Drawing for the job (mm, zero at the part's lowest x, y, z). A direction names the side the tool comes from. Round coordinates to 2 decimals unless told otherwise and drop trailing zeros. Write each loop counter-clockwise with the first axis right and the second up, starting at its lowest first coordinate (ties: lowest second). Pieces come first, ordered by that corner, then holes. Notation, with made-up numbers: M 62,62.25 L 83,62.25 A14 ccw 83,80.25 Z; hole C 81.25,27.25 d6. An arc over 180 degrees is marked long. Use a Markdown table: item, result. Add a question column.
1) Drop flat-ended pins along their axis: P1, Ø2, axis at x = 26.5, y = 25.5, coming from the +Z side; P2, Ø10, axis at y = 15.5, z = 14, coming from the +X side; P3, Ø0.6, axis at y = 23.5, z = 13.5, coming from the -X side. Give the stop position or say it passes through.
2) Slice it at D-D on z = 7.25. Write the cut outline in (x, y).
3) Wall check: probe 1 along Y at (x, z) = (46, 2.5); probe 2 along X at (y, z) = (10, 5.5); probe 3 along X at (y, z) = (15.5, 6.25). Give the ranges that are in metal, low to high.
4) Slice it at B-B on y = 14.25. Write the cut outline in (x, z), plus the area to 3 significant figures.
5) Which spindle directions (+Z, -Z, +X, -X, +Y, -Y) get a long thin tool onto all of the face, cutting with end or side? Do the marked faces 1, 2, 3, 4 and 5. Say none if no direction does.
6) Two-plate mould, pull along X, no slides. Class the marked faces 6, 7 and 8: released by +X, released by -X, zero draft, split by the parting line, or undercut.
7) Slice it at C-C on x = 42. Write the cut outline in (y, z).
8) Slice it at A-A on x = 60. Write the cut outline in (y, z), plus the area to 3 significant figures.
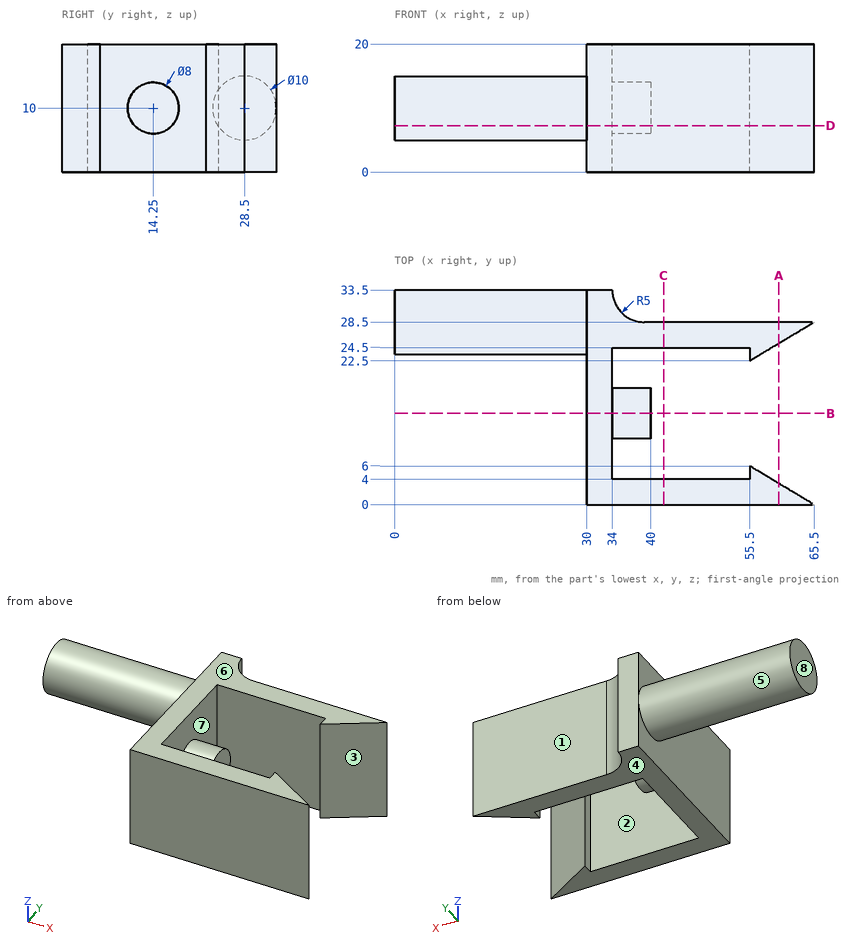
Entries:
| question | item | result |
|---|---|---|
| 1 | P1 | stops at z = 14.58 |
| 1 | P2 | stops at x = 40 |
| 1 | P3 | stops at x = 30 |
| 2 | outline | M 0,24.32 L 30,24.32 L 30,0 L 65.5,0 L 55.5,6 L 55.5,4 L 34,4 L 34,11.35 L 40,11.35 L 40,17.15 L 34,17.15 L 34,24.5 L 55.5,24.5 L 55.5,22.5 L 65.5,28.5 L 39,28.5 A5 cw 34,33.5 L 30,33.5 L 30,32.68 L 0,32.68 Z |
| 3 | probe 1 | y = 0 to 4, 24.5 to 28.5 |
| 3 | probe 2 | x = 30 to 34 |
| 3 | probe 3 | x = 30 to 40 |
| 4 | outline | M 30,0 L 34,0 L 34,6 L 40,6 L 40,14 L 34,14 L 34,20 L 30,20 Z |
| 4 | area | 128 mm^2 |
| 5 | face 1 | +Z, -Z, +X, +Y |
| 5 | face 2 | +Z, -Z |
| 5 | face 3 | +Z, -Z, +X |
| 5 | face 4 | -Z, +X, -X, +Y, -Y |
| 5 | face 5 | -X |
| 6 | face 6 | zero draft |
| 6 | face 7 | undercut |
| 6 | face 8 | released by -X |
| 7 | outline | M 0,0 L 4,0 L 4,20 L 0,20 Z; M 24.5,0 L 28.5,0 L 28.5,20 L 24.5,20 Z |
| 8 | outline | M 0,0 L 3.3,0 L 3.3,20 L 0,20 Z; M 25.2,0 L 28.5,0 L 28.5,20 L 25.2,20 Z |
| 8 | area | 132 mm^2 |
